Verification items for the finished model (mm, model axes). A direction names the side the tool comes from. Coordinates: 2 decimals unless noted, no trailing zeros. Order: outer loops, then holes, each group sorted by start corner. A loop starts at its lowest first (then second) coordinate and runs counter-clockwise, first axis right, second up. Notation, with made-up numbers: M -7.5,28.5 L 47.5,28.5 A15 ccw 47.5,52.5 Z; hole C 60.5,86.5 d1. An arc over 180 degrees is marked long. Return JSON: item names as keys, results as strings.
```python
from build123d import *

# Parameters (mm, degrees)
BOSS_EXTRUDE1_DEPTH = 18
FILLET1_R           = 2
CHAMFER1_SIZE       = 0.6


with BuildPart() as part:
    # Sketch2 → Boss-Extrude1 (new body)
    with BuildSketch(Plane(origin=(-5, 5, -3), x_dir=(0, 1, 0), z_dir=(-1, 0, 0))):
        with BuildLine():
            Line((16.373766646, 1.800474378), (16.687926286, 6.293166529))
            Line((16.687926286, 6.293166529), (7.318960954, 6.948308405))
            ThreePointArc((7.318960954, 6.948308405), (4.926891937, 7.41631163), (2.721626751, 8.45449594))
            ThreePointArc((2.721626751, 8.45449594), (-12.618925504, 0), (2.721626751, -8.45449594))
            ThreePointArc((2.721626751, -8.45449594), (4.926891937, -7.41631163), (7.318960954, -6.948308405))
            Line((7.318960954, -6.948308405), (16.687926286, -6.293166529))
            Line((16.687926286, -6.293166529), (16.373766646, -1.800474378))
            ThreePointArc((16.373766646, -1.800474378), (13.311318022, -1.012179749), (10.388382345, -2.21901322))
            Line((10.388382345, -2.21901322), (10.493272563, -3.71901322))
            Line((10.493272563, -3.71901322), (6.349775255, -4.008754777))
            ThreePointArc((6.349775255, -4.008754777), (3.737837364, -4.547913289), (1.361301465, -5.758280409))
            ThreePointArc((1.361301465, -5.758280409), (-9.618925504, 0), (1.361301465, 5.758280409))
            ThreePointArc((1.361301465, 5.758280409), (3.737837364, 4.547913289), (6.349775255, 4.008754777))
            Line((6.349775255, 4.008754777), (10.493272563, 3.71901322))
            Line((10.493272563, 3.71901322), (10.388382345, 2.21901322))
            ThreePointArc((10.388382345, 2.21901322), (13.311318022, 1.012179749), (16.373766646, 1.800474378))
        make_face()
    extrude(amount=BOSS_EXTRUDE1_DEPTH)

    # Fillet1
    fillet1_edges = [part.edges().sort_by_distance(p)[0] for p in [
        (-14, 21.687926286, 3.293166529),
        (-14, 21.687926286, -9.293166529),
    ]]
    fillet(fillet1_edges, radius=FILLET1_R)

    # Chamfer1
    chamfer1_edges = [part.edges().sort_by_distance(p)[0] for p in [
        (-23, -4.618925504, -3),
        (-23, 8.737837364, -7.547913289),
        (-5, 13.421523909, 0.863883999),
        (-5, 15.440827454, -0.03098678),
        (-5, 18.311318022, -1.987820251),
        (-5, 21.461089992, 0.049256403),
        (-5, 9.926891937, 4.41631163),
        (-5, -7.618925504, -3),
        (-23, 13.421523909, -6.863883999),
        (-5, 9.926891937, -10.41631163),
        (-5, 21.461089992, -6.049256403),
        (-5, 18.311318022, -4.012179749),
        (-5, 15.440827454, -5.96901322),
        (-5, 13.421523909, -6.863883999),
        (-5, 8.737837364, -7.547913289),
        (-5, -4.618925504, -3),
        (-5, 8.737837364, 1.547913289),
        (-23, 15.440827454, -5.96901322),
        (-23, 18.311318022, -4.012179749),
        (-23, 21.461089992, -6.049256403),
        (-23, 9.926891937, -10.41631163),
        (-5, 16.00587957, 3.690493941),
        (-5, 16.00587957, -9.690493941),
        (-5, 21.062704398, -8.749669433),
        (-23, -7.618925504, -3),
        (-5, 21.062704398, 2.749669433),
        (-23, 16.00587957, 3.690493941),
        (-23, 16.00587957, -9.690493941),
        (-23, 21.062704398, -8.749669433),
        (-23, 21.062704398, 2.749669433),
        (-23, 9.926891937, 4.41631163),
        (-23, 8.737837364, 1.547913289),
        (-23, 21.461089992, 0.049256403),
        (-23, 18.311318022, -1.987820251),
        (-23, 15.440827454, -0.03098678),
        (-23, 13.421523909, 0.863883999),
    ]]
    chamfer(chamfer1_edges, length=CHAMFER1_SIZE)


solid = part.part
```
Q1. Go/stop test with flat-tipped pins: pin 1 (3 mm diameter, centred on x = -19.5, y = 6, fed in from -Z); pin 2 (2 mm diameter, centred on y = 11.5, z = -4, fed in from +X). Record where each tip stops, or that it passes through.
Values:
{"pin 1": "z = -12.77", "pin 2": "through"}
Q2. Tool access check on faces 1 (the face through (-22.838, 18.301, -4.452)), 2 (the face through (-5.304, 13.708, -7.14)), 3 (the face through (-13.882, 13.393, -6.866)). Record the directions out of +Z, -Z, +X, -X, +Y, -Y that give a thin tool (end or side, any length) a straight path to the whole face; none if there is none.
Values:
{"face 1": "-X", "face 2": "+X", "face 3": "+X, -X"}
Q3. Draft check along Z on faces 4 (the face through (-13.882, 8.773, 1.536)), 5 (the face through (-22.7, 15.9, 3.4)), 6 (the face through (-5.3, 16.04, -9.39)). Enter one of: pulls with the +Z half, pulls with the -Z half, needs draft (parallel to the pull), parting line crosses it, or undercut.
Values:
{"face 4": "undercut", "face 5": "pulls with the +Z half", "face 6": "pulls with the -Z half"}
Q4. Cross-section at A-A, the plane z = -3. Record the boundary of the cut face in (x, y).
Values:
{"outline": "M -23,-7.02 L -22.4,-7.62 L -5.6,-7.62 L -5,-7.02 L -5,-5.22 L -5.6,-4.62 L -22.4,-4.62 L -23,-5.22 Z"}
Q5. Cross-section at B-B, the plane x = -18.5. Record the boundary of the cut face in (y, z), and give its area (3 significant figures).
Values:
{"outline": "M 6.36,-8.76 A7 cw long 6.36,2.76 A10 ccw 11.35,1.01 L 15.49,0.72 L 15.39,-0.78 A5 ccw 21.37,-1.2 L 21.55,1.3 A2 ccw 19.69,3.43 L 12.32,3.95 A9.9 cw 7.72,5.45 A10 ccw long 7.72,-11.45 A9.9 cw 12.32,-9.95 L 19.69,-9.43 A2 ccw 21.55,-7.3 L 21.37,-4.8 A5 ccw 15.39,-5.22 L 15.49,-6.72 L 11.35,-7.01 A10 ccw Z", "area": "224 mm^2"}
Q6. Material ranges on line 1 along Z through (x, y) = (-16, 2.5); line 2 along Y through (x, z) = (-12.75, -3); line 3 along Y through (x, z) = (-16.5, -6), recorded low to high.
Values:
{"line 1": "-13 to -10, 4 to 7", "line 2": "-7.62 to -4.62", "line 3": "-7.16 to -3.94, 15.44 to 21.46"}
